CAD build for the part. Positions are in the model's coordinates, mm. A direction names the side the tool comes from. Round coordinates to 2 decimals unless told otherwise and drop trailing zeros. Order: outer loops, then holes, each group sorted by start corner. A loop starts at its lowest first (then second) coordinate and runs counter-clockwise, first axis right, second up. Notation, with made-up numbers: (45.25, -25) -> (51.25, -25) arc R15 cw to (51.25, -14) -> close; hole circle Ø3 at (30.5, 5). An arc over 180 degrees is marked (long way). Return JSON: item names as keys, results as strings. Group by question number.
Q1. Probe line 1 along Z through (x, y) = (-1, 16.5); line 2 along Y through (x, z) = (0, 6.5); line 3 along Y through (x, z) = (1, -1). List the from-to ranges inside material, lowest first.
Q2. Cut at A-A (y = 18). Write the cut outline in (x, z).
Q3. Cut at B-B (x = 0). Count the separate pieces of the cut face and the enclosed holes in it, then the cut area to 3 significant figures.
Q4. Flat gauge pins, fed straight in: pin 1 (2 mm diameter, centred on y = -3.5, z = 1, fed in from -X); pin 2 (2.5 mm diameter, centred on x = 10.59, y = 10.62, fed in from +Z); pin 3 (1.5 mm diameter, centred on y = -2.5, z = -2, fed in from -X); pin 4 (1 mm diameter, centred on y = 0.5, z = 3, fed in from -X). Where does each tip first touch, or does it go through?
Q5. Which spindle directions (+Z, -Z, +X, -X, +Y, -Y) get a long thin tool onto all of the face, cutting with end or side? Do faces 1 (the cylindrical face through (11.98, 10.05, 9.02)), 2 (the flat face through (10, -10, 2.246)). Say none if no direction does.
Q6. Mould opens along X. For faces 3 (the cylindrical face through (-0.867, -3.905, 1.258)), 4 (the cylindrical face through (10.382, -19.961, 1.107)), 5 (the flat face through (10, -10, 0)) say: +X half, -X half, draft (parallel to the pull), parting line (faces both ways), or undercut.
Q7. Cut at D-D (x = -16). Write the cut outline in (y, z), then the cut area to 3 significant figures.
from build123d import *

# Parameters (mm, degrees)
SKETCH1_R           = 22.5
BOSS_EXTRUDE1_DEPTH = 2.24600008
SKETCH2_R           = 13
BOSS_EXTRUDE2_DEPTH = 5
BOSS_EXTRUDE4_START = 3.5
SKETCH5_R           = 22.5
BOSS_EXTRUDE4_DEPTH = 3.5
BOSS_EXTRUDE5_START = 5
SKETCH8_R           = 13
BOSS_EXTRUDE5_DEPTH = 5
SKETCH12_R          = 22.5
BOSS_EXTRUDE6_DEPTH = 3.5
SKETCH6_R           = 4
SKETCH6_R_2         = 2.15
SKETCH6_R_3         = 1.5
CUT_EXTRUDE1_DEPTH  = 38.187477988


with BuildPart() as part:
    # Sketch1 → Boss-Extrude1 (new body)
    with BuildSketch(Plane.XY):
        Circle(SKETCH1_R)
    extrude(amount=BOSS_EXTRUDE1_DEPTH)

    # Sketch2 → Boss-Extrude2 (add)
    with BuildSketch(Plane.XY):
        Circle(SKETCH2_R)
    extrude(amount=-BOSS_EXTRUDE2_DEPTH)

    # Sketch5 → Boss-Extrude4 (add)
    with BuildSketch(Plane(origin=(0, 0, -5), x_dir=(-1, 0, 0), z_dir=(0, 0, -1)).offset(BOSS_EXTRUDE4_START)):
        with Locations(Location((0, 0, 0), (0, 0, 180))):
            Circle(SKETCH5_R)
    extrude(amount=-BOSS_EXTRUDE4_DEPTH)

    # Sketch8 → Boss-Extrude5 (add)
    with BuildSketch(Plane.XY.offset(2.24600008).offset(BOSS_EXTRUDE5_START)):
        Circle(SKETCH8_R)
    extrude(amount=-BOSS_EXTRUDE5_DEPTH)

    # Sketch12 → Boss-Extrude6 (add)
    with BuildSketch(Plane.XY.offset(7.24600008)):
        Circle(SKETCH12_R)
    extrude(amount=BOSS_EXTRUDE6_DEPTH)

    # Sketch6 → Cut-Extrude1 (cut, through all)
    with BuildSketch(Plane.XY.offset(10.74600008)):
        Circle(SKETCH6_R)
        with Locations((0, 9.779)):
            Circle(SKETCH6_R_2)
        with Locations((9.779, 0)):
            Circle(SKETCH6_R_2)
        with Locations((0, -9.779)):
            Circle(SKETCH6_R_2)
        with Locations((-9.779, 0)):
            Circle(SKETCH6_R_2)
        with Locations((10.592506585, 10.620678145)):
            Circle(SKETCH6_R_3)
        with Locations((13.586186135, 6.35732226)):
            Circle(SKETCH6_R_3)
    extrude(amount=-CUT_EXTRUDE1_DEPTH, mode=Mode.SUBTRACT)


solid = part.part
Solution:
{
 "1": {"line 1": "z = -8.5 to -5, 0 to 2.25, 7.25 to 10.75", "line 2": "y = -13 to -11.93, -7.63 to -4, 4 to 7.63, 11.93 to 13", "line 3": "y = -12.96 to -11.68, -7.88 to -3.87, 3.87 to 7.88, 11.68 to 12.96"},
 "2": {"outline": "(-13.5, -8.5) -> (13.5, -8.5) -> (13.5, -5) -> (-13.5, -5) -> close; (-13.5, 0) -> (13.5, 0) -> (13.5, 2.25) -> (-13.5, 2.25) -> close; (-13.5, 7.25) -> (13.5, 7.25) -> (13.5, 10.75) -> (-13.5, 10.75) -> close"},
 "3": {"separate pieces": "4", "enclosed holes": "0", "area": "357 mm²"},
 "4": {"pin 1": "stops at x = -22.36", "pin 2": "passes through", "pin 3": "stops at x = -12.88", "pin 4": "stops at x = -13"},
 "5": {"face 1": "+Z, -Z", "face 2": "none"},
 "6": {"face 3": "undercut", "face 4": "parting line", "face 5": "draft"},
 "7": {"outline": "(-15.82, -8.5) -> (15.82, -8.5) -> (15.82, -5) -> (-15.82, -5) -> close; (-15.82, 0) -> (15.82, 0) -> (15.82, 2.25) -> (-15.82, 2.25) -> close; (-15.82, 7.25) -> (15.82, 7.25) -> (15.82, 10.75) -> (-15.82, 10.75) -> close", "area": "293 mm²"}
}
